Geometry: see drawing. Coordinates: mm, zero at the bounding-box minimum. A direction names the side the tool comes from. Round coordinates to 2 decimals unless told otherwise and drop trailing zeros. Order: outer loops, then holes, each group sorted by start corner. A loop starts at its lowest first (then second) coordinate and runs counter-clockwise, first axis right, second up. Notation, with made-up numbers: (41.5, 74.25) -> (77.5, 74.25) arc R33 ccw to (77.5, 104.25) -> close; hole circle Ø7 at (31, 49.25). An arc over 180 degrees is marked (long way). Put each result on its own line as item: value.
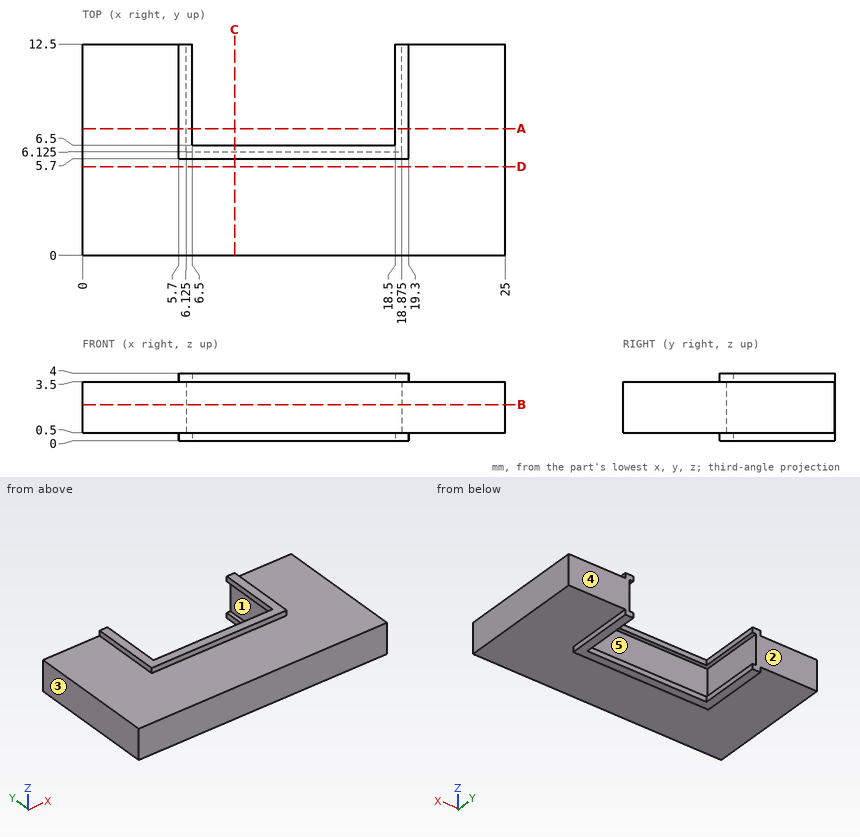
1. Cut plane D-D on y = 5.25. Return loops of the section in (x, z).
Ans:
outline: (0, 0.5) -> (25, 0.5) -> (25, 3.5) -> (0, 3.5) -> close
2. Material intervals for probe 1 along X at (y, z) = (6.5, 2.6) (3 decimals); probe 2 along Z at (x, y) = (5.75, 0.5); probe 3 along Y at (x, z) = (12.75, 0.25), sorted ascending.
Ans:
probe 1: 0 to 6.125, 18.875 to 25
probe 2: 0.5 to 3.5
probe 3: 5.7 to 6.5
3. Set-up query: the marked faces 1 and 2. Return all of +Z, -Z, +X, -X, +Y, -Y with unobstructed straight access to the full face (end or side cutting, diameter ignored); none if empty.
Ans:
face 1: +Y
face 2: +Z, -Z, +X, -X, +Y
4. Contact query for flat-ended pins moving along their axis: P1, Ø0.6, axis at y = 8, z = 4, coming from the +X side; P2, Ø0.6, axis at x = 15, z = 3.5, coming from the -Y side; P3, Ø0.6, axis at y = 8.5, z = 0, coming from the -X side; P4, Ø2, axis at x = 17, y = 1.5, coming from the -Z side. Output: stop coordinate, or through.
Ans:
P1: x = 19.3
P2: y = 0
P3: x = 5.7
P4: z = 0.5
5. Cut plane A-A on y = 7.5. Return loops of the section in (x, z) (3 decimals), and give its area (4 significant figures).
Ans:
outline: (0, 0.5) -> (5.7, 0.5) -> (5.7, 0) -> (6.5, 0) -> (6.5, 0.5) -> (6.125, 0.5) -> (6.125, 3.5) -> (6.5, 3.5) -> (6.5, 4) -> (5.7, 4) -> (5.7, 3.5) -> (0, 3.5) -> close; (18.5, 0) -> (19.3, 0) -> (19.3, 0.5) -> (25, 0.5) -> (25, 3.5) -> (19.3, 3.5) -> (19.3, 4) -> (18.5, 4) -> (18.5, 3.5) -> (18.875, 3.5) -> (18.875, 0.5) -> (18.5, 0.5) -> close
area: 38.35 mm²
6. Draft query along X for the marked faces 3, 4 and 5. Return one class per face: +X half, -X half, draft (parallel to the pull), parting line (faces both ways), or undercut.
Ans:
face 3: -X half
face 4: draft
face 5: undercut
7. Cut plane B-B on z = 2.15. Return loops of the section in (x, y) (3 decimals), and give its area (3 significant figures).
Ans:
outline: (0, 0) -> (25, 0) -> (25, 12.5) -> (18.875, 12.5) -> (18.875, 6.125) -> (6.125, 6.125) -> (6.125, 12.5) -> (0, 12.5) -> close
area: 231 mm²
8. Cut plane C-C on x = 9. Return loops of the section in (y, z) (3 decimals).
Ans:
outline: (0, 0.5) -> (5.7, 0.5) -> (5.7, 0) -> (6.5, 0) -> (6.5, 0.5) -> (6.125, 0.5) -> (6.125, 3.5) -> (6.5, 3.5) -> (6.5, 4) -> (5.7, 4) -> (5.7, 3.5) -> (0, 3.5) -> close
